Can you work these out from the drawing? Everything is in mm from the part's minimum corner. A direction names the side the tool comes from. Coordinates: 2 decimals unless noted, no trailing zeros. Order: outer loops, then holes, each group sorted by start corner. A loop starts at its lowest first (then second) coordinate and runs counter-clockwise, first axis right, second up. Notation, with made-up numbers: (68.25, 69.5) - (79.25, 69.5) arc R15 ccw to (79.25, 75.5) - close; hole circle Ø1 at (-14, 57.5). An arc over 180 degrees is marked (long way). Answer as CSV lines item,"result". Start each with the question number.
Q1. For pin 1 Ø9 at (x, z) = (5.5, 9.5) entering from -Y; pin 2 Ø1.5 at (x, y) = (11.5, 16) entering from +Z; pin 3 Ø4 at (x, z) = (33.5, 6) entering from +Y, each with a flat end and sliding along its axis, tell me the tip position at first contact or that it passes through.
Q2. Suppose I cut it at A-A (z = 14). Please give me the cut outline in (x, y).
Q3. Thinking about a two-plate mould opening in X: for the marked faces 4, 5 and 6, which applies, released by +X, released by -X, zero draft, split by the parting line, or undercut?
Q4. Suppose I cut it at C-C (z = 9.1). Please give me the cut outline in (x, y).
Q5. Suppose I cut it at B-B (y = 10.1). Please give me the cut outline in (x, z).
Q6. I need wall thicknesses on line 1 (X direction, y = 20.8, z = 9.1); line 2 (X direction, y = 10.1, z = 0.1); line 3 (Y direction, x = 38.5, z = 0.4). Which ranges of each line are inside material? Lowest first, please.
Q7. For the marked faces 1, 2 and 3, which set-ups out of +Z, -Z, +X, -X, +Y, -Y let a thin tool reach every point of the face, with its end or its side?
Q8. Suppose I cut it at D-D (x = 6.5). Please give me the cut outline in (y, z), then the cut area to 3 significant figures.
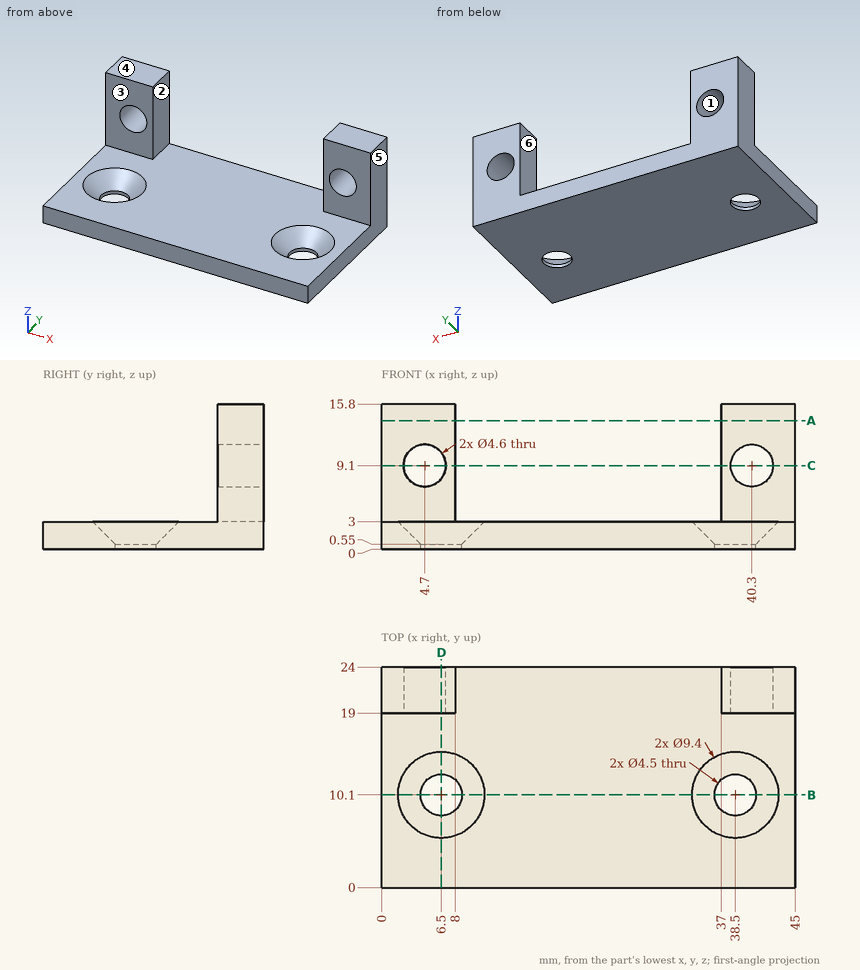
Here are the results:
1,pin 1,"stops at y = 19"
1,pin 2,"stops at z = 3"
1,pin 3,"passes through"
2,outline,"(0, 19) - (8, 19) - (8, 24) - (0, 24) - close; (37, 19) - (45, 19) - (45, 24) - (37, 24) - close"
3,face 4,"zero draft"
3,face 5,"released by +X"
3,face 6,"undercut"
4,outline,"(0, 19) - (2.4, 19) - (2.4, 24) - (0, 24) - close; (7, 19) - (8, 19) - (8, 24) - (7, 24) - close; (37, 19) - (38, 19) - (38, 24) - (37, 24) - close; (42.6, 19) - (45, 19) - (45, 24) - (42.6, 24) - close"
5,outline,"(0, 0) - (4.25, 0) - (4.25, 0.55) - (1.8, 3) - (0, 3) - close; (8.75, 0) - (36.25, 0) - (36.25, 0.55) - (33.8, 3) - (11.2, 3) - (8.75, 0.55) - close; (40.75, 0) - (45, 0) - (45, 3) - (43.2, 3) - (40.75, 0.55) - close"
6,line 1,"x = 0 to 2.4, 7 to 8, 37 to 38, 42.6 to 45"
6,line 2,"x = 0 to 4.25, 8.75 to 36.25, 40.75 to 45"
6,line 3,"y = 0 to 7.85, 12.35 to 24"
7,face 1,"+Y, -Y"
7,face 2,"+Z, +Y, -Y"
7,face 3,"+Z, +X, -X, -Y"
8,outline,"(0, 0) - (7.85, 0) - (7.85, 0.55) - (5.4, 3) - (0, 3) - close; (12.35, 0) - (24, 0) - (24, 7.67) - (19, 7.67) - (19, 3) - (14.8, 3) - (12.35, 0.55) - close; (19, 10.53) - (24, 10.53) - (24, 15.8) - (19, 15.8) - close"
8,area,"102 mm²"
